from build123d import *

# Parameters (mm, degrees)
SKETCH_R        = 13
PAD_DEPTH       = 7
SKETCH001_R     = 3
PAD001_DEPTH    = 3
CHAMFER_SIZE    = 1
SKETCH002_R     = 25
PAD002_DEPTH    = 3
CHAMFER001_SIZE = 3


with BuildPart() as part:
    # Sketch → Pad (new body)
    with BuildSketch(Plane.XY):
        Circle(SKETCH_R)
    extrude(amount=PAD_DEPTH)

    # Sketch001 (on Face3 of Pad) → Pad001 (join)
    with BuildSketch(Plane.XY.offset(7)):
        with Locations((-6.5, 6.5)):
            Circle(SKETCH001_R)
        with Locations((-6.5, -6.5)):
            Circle(SKETCH001_R)
        with Locations((6.5, -6.5)):
            Circle(SKETCH001_R)
        with Locations((6.5, 6.5)):
            Circle(SKETCH001_R)
    extrude(amount=PAD001_DEPTH)

    # Chamfer
    chamfer_edges = [part.edges().sort_by_distance(p)[0] for p in [
        (-9.5, -6.5, 10),
        (3.5, -6.5, 10),
        (-9.5, 6.5, 10),
        (3.5, 6.5, 10),
    ]]
    chamfer(chamfer_edges, length=CHAMFER_SIZE)

    # Sketch002 (on Face9 of Chamfer) → Pad002 (join)
    with BuildSketch(Plane(origin=(0, 0, 0), x_dir=(1, 0, 0), z_dir=(0, 0, -1))):
        Circle(SKETCH002_R)
    extrude(amount=PAD002_DEPTH)

    # Chamfer001
    chamfer001_edges = [part.edges().sort_by_distance(p)[0] for p in [
        (-13, 0, 0),
    ]]
    chamfer(chamfer001_edges, length=CHAMFER001_SIZE)


solid = part.part
Work out the finished part from the listing and answer in its coordinate system (mm). A direction names the side the tool comes from. Coordinates: 2 decimals unless noted, no trailing zeros. Loops run counter-clockwise (first coordinate to the right, second up) from the corner with the lowest first, then second, coordinate; pieces in that order, holes last. Notation, with made-up numbers: (60, 7) -> (80, 7) arc R6 cw to (80, 11) -> close; hole circle Ø5 at (43, -32). An arc over 180 degrees is marked (long way). Answer as CSV lines item,"result".
1) The part is cut by section A-A (y = 0). Give the vertices of the cut face in (x, z).
A:
outline,"(-25, -3) -> (25, -3) -> (25, 0) -> (16, 0) -> (13, 3) -> (13, 7) -> (-13, 7) -> (-13, 3) -> (-16, 0) -> (-25, 0) -> close"
2) The part is cut by section D-D (y = -21). Give the vertices of the cut face in (x, z), and give its area (3 significant figures).
A:
outline,"(-13.56, -3) -> (13.56, -3) -> (13.56, 0) -> (-13.56, 0) -> close"
area,"81.4 mm²"
3) Straight lines are drawn through the part: probe 1 along Z at (x, y) = (-6, -0.5); probe 2 along X at (y, z) = (0.5, 6); probe 3 along Z at (x, y) = (22, 6). For each, find the intervals that lie inside material, in ascending order.
A:
probe 1,"z = -3 to 7"
probe 2,"x = -12.99 to 12.99"
probe 3,"z = -3 to 0"
4) The part is cut by section C-C (y = 17). Give the vertices of the cut face in (x, z).
A:
outline,"(-18.33, -3) -> (18.33, -3) -> (18.33, 0) -> (-18.33, 0) -> close"
5) Flat-ended cylindrical pins translate along their axes: pin 1 (6 mm diameter, centred on x = 16.5, z = -0.5, fed in from +Y); pin 2 (2 mm diameter, centred on x = -5.5, z = 7, fed in from -Y); pin 3 (8 mm diameter, centred on x = 1, y = -4, fed in from +Z). Find the tip coordinate at first contact, or state that the pin passes through.
A:
pin 1,"stops at y = 21.04"
pin 2,"stops at y = -12.2"
pin 3,"stops at z = 9.96"
6) For a pull along X with two mould halves and no side action, classify faces 3 (the face through (0, 0, 7)), 4 (the face through (0, 0, -3)), 5 (the face through (-10.316, -7.91, 4.972)) as released by +X, released by -X, zero draft, split by the parting line, or undercut.
A:
face 3,"undercut"
face 4,"zero draft"
face 5,"split by the parting line"
7) For faces 1 (the face through (23.846, -7.509, -1.479)), 2 (the face through (-3.73, 5.35, 7.99)), determine the directions among +Z, -Z, +X, -X, +Y, -Y from which every point of the face is accessible in a straight line to the end or side of a thin tool.
A:
face 1,"+Z, -Z"
face 2,"+Z"
